The figure shows three views and two pictorial views of one solid part (mm, origin at its lowest corner). Answer the questions. A direction names the side the tool comes from. Coordinates: 2 decimals unless noted, no trailing zeros. Loops run counter-clockwise (first coordinate to the right, second up) from the corner with the lowest first, then second, coordinate; pieces in that order, holes last. Notation, with made-up numbers: M 85,12.25 L 117,12.25 A21 cw 117,29.25 Z; hole C 43,81.5 d11. An arc over 180 degrees is marked long. Answer as a JSON object with one key per item and string values. Group by question number.
1. Straight lines are drawn through the part: L1, parallel to X at y = 3, z = 55; L2, parallel to Y at x = 18.5, z = 91.5; L3, parallel to Y at x = 97, z = 50. For each, find the intervals that lie inside material, in ascending order.
2. A cutting plane is placed at B-B on z = 55. Give the vertices of the cut face in (x, y), and give its area (3 significant figures).
3. A cutting plane is placed at C-C on y = 3. Give the vertices of the cut face in (x, z).
4. For the marked faces 4, 5 and 6, determine the directions among +Z, -Z, +X, -X, +Y, -Y from which every point of the face is accessible in a straight line to the end or side of a thin tool.
5. Determine the mould class of the marked faces 1, 2 and 3 for opening direction Y: released by +Y, released by -Y, zero draft, split by the parting line, or undercut.
6. A cutting plane is placed at A-A on x = 55. Give the vertices of the cut face in (y, z).
7. Given pin 1 (1 mm diameter, centred on x = 38.5, y = 46, fed in from +Z); pin 2 (5 mm diameter, centred on y = 22.5, z = 33, fed in from +X); pin 3 (11 mm diameter, centred on x = 21.5, y = 28.5, fed in from -Z); pin 4 (12 mm diameter, centred on x = 43, z = 82.5, fed in from -Y), each flat-ended and moving along its own axis, determine where each tip first touches the part or whether it passes through.
8. A cutting plane is placed at D-D on z = 20. Give the vertices of the cut face in (x, y), and give its area (3 significant figures).
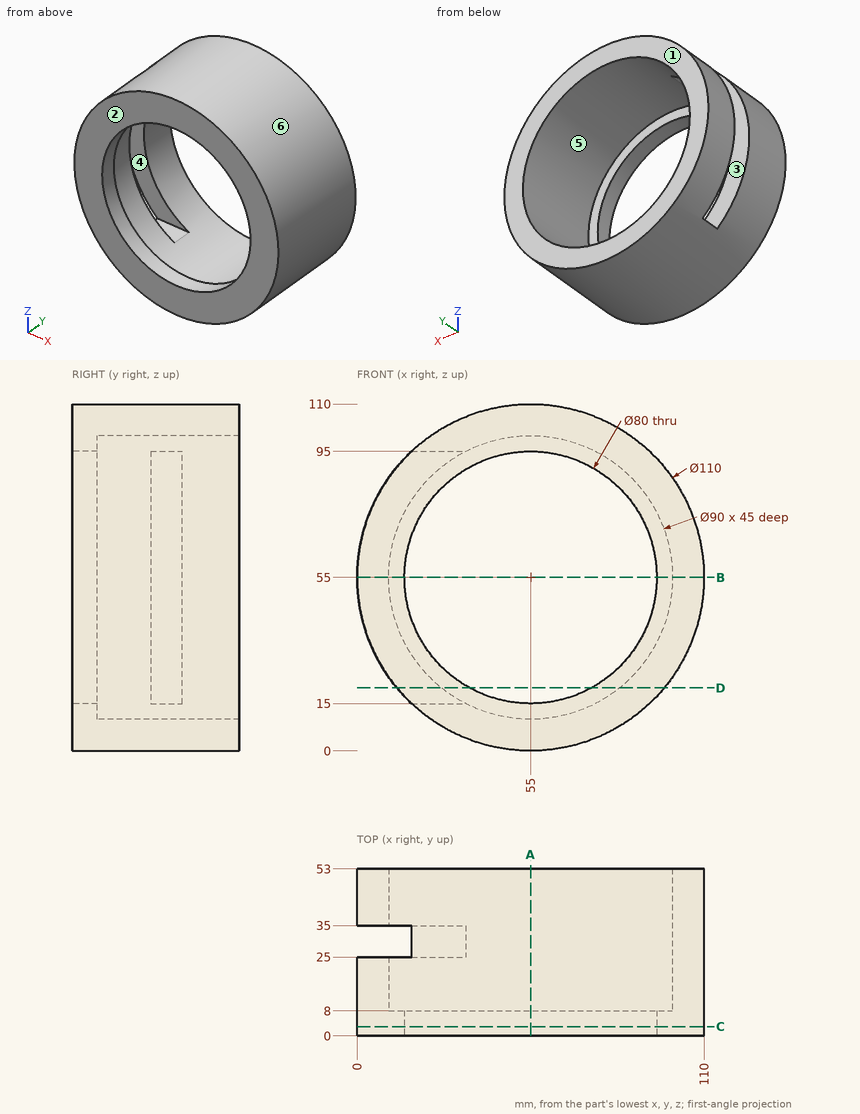
From the geometry:
{
 "1": {"L1": "x = 0 to 15, 95 to 110", "L2": "y = 0 to 25, 35 to 53", "L3": "y = 0 to 8"},
 "2": {"outline": "M 0,0 L 15,0 L 15,8 L 10,8 L 10,25 L 0,25 Z; M 0,35 L 10,35 L 10,53 L 0,53 Z; M 95,0 L 110,0 L 110,53 L 100,53 L 100,8 L 95,8 Z", "area": "1,040 mm²"},
 "3": {"outline": "C 55,55 d110; hole C 55,55 d80"},
 "4": {"face 4": "-X", "face 5": "+Y", "face 6": "+Y, -Y"},
 "5": {"face 1": "released by +Y", "face 2": "released by -Y", "face 3": "undercut"},
 "6": {"outline": "M 0,0 L 53,0 L 53,10 L 8,10 L 8,15 L 0,15 Z; M 0,95 L 8,95 L 8,100 L 53,100 L 53,110 L 0,110 Z"},
 "7": {"pin 1": "stops at z = 107.62", "pin 2": "stops at x = 106.43", "pin 3": "stops at z = 7.66", "pin 4": "passes through"},
 "8": {"outline": "M 12.57,0 L 35.64,0 L 35.64,8 L 26.72,8 L 26.72,25 L 12.57,25 Z; M 12.57,35 L 26.72,35 L 26.72,53 L 12.57,53 Z; M 74.36,0 L 97.43,0 L 97.43,53 L 83.28,53 L 83.28,8 L 74.36,8 Z", "area": "1,500 mm²"}
}
